Part model, mm, in its own coordinate system. Give positions to 0.01 mm unless a question says otherwise; leave off trailing zeros. Write each loop counter-clockwise with the first axis right and the second up, starting at its lowest first coordinate (ties: lowest second). Pieces come first, ordered by that corner, then holes.
from build123d import *

# Parameters (mm, degrees)
SKETCH1_W           = 50
SKETCH1_H           = 25
SKETCH1_R           = 4.65
SKETCH1_R_2         = 1.75
SKETCH1_R_3         = 2
BOSS_EXTRUDE1_DEPTH = 3.385


with BuildPart() as part:
    # Sketch1 → Boss-Extrude1 (new body)
    with BuildSketch(Plane.XY):
        Rectangle(SKETCH1_W, SKETCH1_H)
        Circle(SKETCH1_R, mode=Mode.SUBTRACT)
        with Locations((-10, 0)):
            Circle(SKETCH1_R_2, mode=Mode.SUBTRACT)
        with Locations((20, 0)):
            Circle(SKETCH1_R_3, mode=Mode.SUBTRACT)
        with Locations((-20, 0)):
            Circle(SKETCH1_R_3, mode=Mode.SUBTRACT)
    extrude(amount=BOSS_EXTRUDE1_DEPTH)


solid = part.part
1) Saw through at C-C (x = 0). Write the cut outline in (y, z) (3 decimals), and give its area (3 significant figures).
Check result:
outline: (-12.5, 0) - (-4.65, 0) - (-4.65, 3.385) - (-12.5, 3.385) - close; (4.65, 0) - (12.5, 0) - (12.5, 3.385) - (4.65, 3.385) - close
area: 53.1 mm2
2) Mould opens along X. For faces 1 (the cylindrical face through (2.5, 3.92, 1.67)), 2 (the flat face through (25, 0, 2)), 3 (the flat face through (-6, 0, 0)) say: +X half, -X half, draft (parallel to the pull), parting line (faces both ways), or undercut.
Check result:
face 1: undercut
face 2: +X half
face 3: draft
3) Saw through at A-A (x = -20). Write the cut outline in (y, z) (3 decimals).
Check result:
outline: (-12.5, 0) - (-2, 0) - (-2, 3.385) - (-12.5, 3.385) - close; (2, 0) - (12.5, 0) - (12.5, 3.385) - (2, 3.385) - close
4) Flat gauge pin, fed straight in: P1, Ø3, axis at x = -10, y = 0, coming from the +Z side. Where does the tip first touch, or does it go through?
Check result:
P1: passes through
5) Saw through at B-B (z = 2.9). Write the cut outline in (x, y), and give its area (3 significant figures).
Check result:
outline: (-25, -12.5) - (25, -12.5) - (25, 12.5) - (-25, 12.5) - close; hole circle Ø4 at (-20, 0); hole circle Ø3.5 at (-10, 0); hole circle Ø9.3 at (0, 0); hole circle Ø4 at (20, 0)
area: 1,150 mm2
6) Drill centre lines: L1, parallel to Y at x = 20, z = 1.05; L2, parallel to Y at x = -10, z = 1.4; L3, parallel to X at y = -3.5, z = 0.55. Where is each one in solid material? Low to high.
Check result:
L1: y = -12.5 to -2, 2 to 12.5
L2: y = -12.5 to -1.75, 1.75 to 12.5
L3: x = -25 to -3.06, 3.06 to 25
